For this review, take the finished solid that the model builds, in its own axes (mm). Round coordinates to 2 decimals unless told otherwise and drop trailing zeros. Put each result on its own line as item: value.
from build123d import *

# Parameters (mm, degrees)
SKETCH1_W           = 270
SKETCH1_H           = 200
SKETCH1_R           = 1.5
SKETCH1_R_2         = 10
SKETCH1_W_2         = 4
SKETCH1_H_2         = 20
BOSS_EXTRUDE1_DEPTH = 4


with BuildPart() as part:
    # Sketch1 → Boss-Extrude1 (new body)
    with BuildSketch(Plane.XY):
        with Locations((71.763348527, -16.133333333)):
            Rectangle(SKETCH1_W, SKETCH1_H)
        with Locations((-35.236651473, -92.133333333)):
            Circle(SKETCH1_R, mode=Mode.SUBTRACT)
        with Locations((-20.236651473, -92.133333333)):
            Circle(SKETCH1_R, mode=Mode.SUBTRACT)
        with Locations((-35.236651473, -107.133333333)):
            Circle(SKETCH1_R, mode=Mode.SUBTRACT)
        with Locations((-50.236651473, -92.133333333)):
            Circle(SKETCH1_R, mode=Mode.SUBTRACT)
        with Locations((-35.236651473, -77.133333333)):
            Circle(SKETCH1_R, mode=Mode.SUBTRACT)
        with Locations((71.763348527, -16.133333333)):
            Circle(SKETCH1_R, mode=Mode.SUBTRACT)
        with Locations((193.763348527, -92.133333333)):
            Circle(SKETCH1_R, mode=Mode.SUBTRACT)
        with Locations((178.763348527, -77.133333333)):
            Circle(SKETCH1_R, mode=Mode.SUBTRACT)
        with Locations((178.763348527, -92.133333333)):
            Circle(SKETCH1_R, mode=Mode.SUBTRACT)
        with Locations((178.763348527, -107.133333333)):
            Circle(SKETCH1_R, mode=Mode.SUBTRACT)
        with Locations((163.763348527, -92.133333333)):
            Circle(SKETCH1_R, mode=Mode.SUBTRACT)
        with Locations((193.763348527, 59.866666667)):
            Circle(SKETCH1_R, mode=Mode.SUBTRACT)
        with Locations((178.763348527, 74.866666667)):
            Circle(SKETCH1_R, mode=Mode.SUBTRACT)
        with Locations((178.763348527, 59.866666667)):
            Circle(SKETCH1_R, mode=Mode.SUBTRACT)
        with Locations((178.763348527, 44.866666667)):
            Circle(SKETCH1_R, mode=Mode.SUBTRACT)
        with Locations((163.763348527, 59.866666667)):
            Circle(SKETCH1_R, mode=Mode.SUBTRACT)
        with Locations((-20.236651473, 59.866666667)):
            Circle(SKETCH1_R, mode=Mode.SUBTRACT)
        with Locations((-35.236651473, 74.866666667)):
            Circle(SKETCH1_R, mode=Mode.SUBTRACT)
        with Locations((-35.236651473, 59.866666667)):
            Circle(SKETCH1_R, mode=Mode.SUBTRACT)
        with Locations((-35.236651473, 44.866666667)):
            Circle(SKETCH1_R, mode=Mode.SUBTRACT)
        with Locations((-50.236651473, 59.866666667)):
            Circle(SKETCH1_R, mode=Mode.SUBTRACT)
        with Locations((178.763348527, -16.133333333)):
            Circle(SKETCH1_R, mode=Mode.SUBTRACT)
        with Locations((95.763348527, 18.866666667)):
            Circle(SKETCH1_R, mode=Mode.SUBTRACT)
        with Locations((71.763348527, 59.866666667)):
            Circle(SKETCH1_R, mode=Mode.SUBTRACT)
        with Locations((16.763348527, 59.866666667)):
            Circle(SKETCH1_R_2, mode=Mode.SUBTRACT)
        with Locations((16.763348527, -92.133333333)):
            Circle(SKETCH1_R_2, mode=Mode.SUBTRACT)
        with Locations((-35.236651473, -16.133333333)):
            Circle(SKETCH1_R, mode=Mode.SUBTRACT)
        with Locations((71.763348527, -92.133333333)):
            Circle(SKETCH1_R, mode=Mode.SUBTRACT)
        with Locations((26.763348527, -70.133333333)):
            Circle(SKETCH1_R, mode=Mode.SUBTRACT)
        with Locations((-27.236651473, -16.133333333)):
            Circle(SKETCH1_R, mode=Mode.SUBTRACT)
        with Locations((26.763348527, 37.866666667)):
            Circle(SKETCH1_R, mode=Mode.SUBTRACT)
        with Locations((80.763348527, -16.133333333)):
            Circle(SKETCH1_R, mode=Mode.SUBTRACT)
        with Locations((147.763348527, 18.866666667)):
            Circle(SKETCH1_R, mode=Mode.SUBTRACT)
        with Locations((147.763348527, -51.133333333)):
            Circle(SKETCH1_R, mode=Mode.SUBTRACT)
        with Locations((95.763348527, -51.133333333)):
            Circle(SKETCH1_R, mode=Mode.SUBTRACT)
        with Locations((-3.236651473, 35.366666667)):
            Circle(SKETCH1_R, mode=Mode.SUBTRACT)
        with Locations((54.763348527, 35.366666667)):
            Circle(SKETCH1_R, mode=Mode.SUBTRACT)
        with Locations((54.763348527, -67.633333333)):
            Circle(SKETCH1_R, mode=Mode.SUBTRACT)
        with Locations((-3.236651473, -67.633333333)):
            Circle(SKETCH1_R, mode=Mode.SUBTRACT)
        with Locations((-51.236651473, 43.866666667)):
            Rectangle(SKETCH1_W_2, SKETCH1_H_2, mode=Mode.SUBTRACT)
        with Locations((-51.236651473, -76.133333333)):
            Rectangle(SKETCH1_W_2, SKETCH1_H_2, mode=Mode.SUBTRACT)
    extrude(amount=BOSS_EXTRUDE1_DEPTH)


solid = part.part
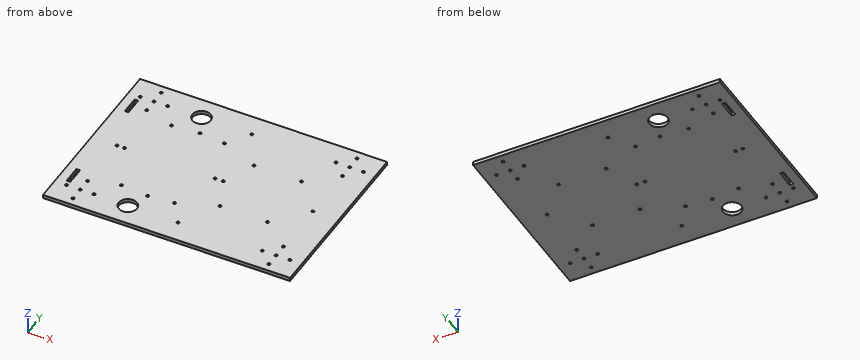
(1) Insertion check: pin 1 Ø2.5 at (x, y) = (-20.24, 59.87) entering from +Z. The pin has a flat end and moves straight along its axis. Give the tip position at first contact, or say it passes through.
A:
pin 1: passes through
(2) Add section A-A on z = 1. State how many separate pieces and enclosed holes the cut face has, then the cut area to 4 significant figures.
A:
separate pieces: 1
enclosed holes: 41
area: 52,950 mm2
(3) To check wall thickness, follow L1, parallel to X at y = 18.5, z = 1.4; L2, parallel to X at y = 37.5, z = 1.7; L3, parallel to Y at x = 165, z = 3.1. State the ranges of each line that lie inside material, in increasing order.
A:
L1: x = -63.24 to 94.31, 97.22 to 146.31, 149.22 to 206.76
L2: x = -63.24 to -53.24, -49.24 to 25.31, 28.22 to 206.76
L3: y = -116.13 to -92.98, -91.28 to 59.02, 60.72 to 83.87
